Check sheet for the modelled part. Datum: model origin and axes. Units: mm. Coordinates: 2 decimals unless noted, no trailing zeros. Loops run counter-clockwise (first coordinate to the right, second up) from the corner with the lowest first, then second, coordinate; pieces in that order, holes last. Notation, with made-up numbers: M 21,56 L 80,56 A24 cw 80,72 Z; hole C -22,11 d9. An arc over 180 degrees is marked long. Return JSON: item names as keys, results as strings.
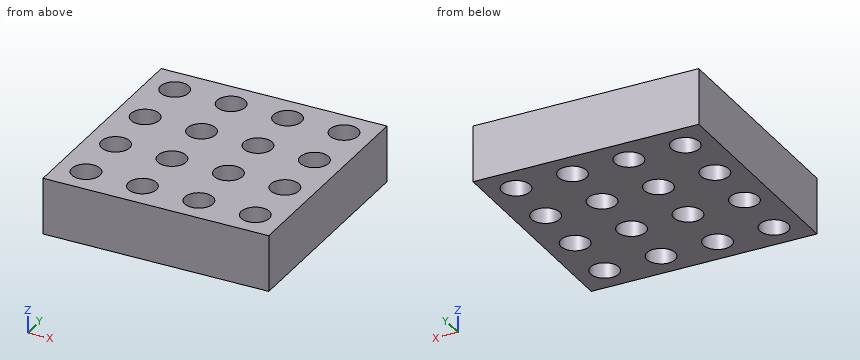
from build123d import *

# Parameters (mm, degrees)
SKETCH1_W            = 40
SKETCH1_H            = 40
BOSS_EXTRUDE1_DEPTH  = 10
SKETCH3_R            = 2.5
CUT_EXTRUDE1_DEPTH   = 11
LPATTERN1_COUNT      = 4
LPATTERN1_PITCH      = 10
LPATTERN1_COUNT_DIR2 = 4
LPATTERN1_PITCH_DIR2 = 10


with BuildPart() as part:
    # Sketch1 → Boss-Extrude1 (new body)
    with BuildSketch(Plane.XY):
        Rectangle(SKETCH1_W, SKETCH1_H)
    extrude(amount=BOSS_EXTRUDE1_DEPTH)

    # Sketch3 → Cut-Extrude1 (cut, through all)
    with BuildSketch(Plane.XY.offset(10)):
        with Locations((15, 15)):
            Circle(SKETCH3_R)
    cut_extrude1 = extrude(amount=-CUT_EXTRUDE1_DEPTH, mode=Mode.SUBTRACT)

    # LPattern1: Cut-Extrude1 4 × 4
    with Locations(*[(-i * LPATTERN1_PITCH, -j * LPATTERN1_PITCH_DIR2, 0) for i in range(LPATTERN1_COUNT) for j in range(LPATTERN1_COUNT_DIR2) if (i, j) != (0, 0)]):
        add(cut_extrude1, mode=Mode.SUBTRACT)


solid = part.part
1) Section check B-B on z = 3.25. Count the separate pieces of the cut face and the enclosed holes in it, then the cut area to 3 significant figures.
Answers:
{"separate pieces": "1", "enclosed holes": "16", "area": "1,290 mm²"}
2) Scan lines: line 1 along Y through (x, z) = (5, 6); line 2 along Y through (x, z) = (4, 2.5); line 3 along X through (y, z) = (-13, 4.5). Record each from-to range of solid material in increasing order. Write a range as [from, to].
Answers:
{"line 1": "[-20, -17.5], [-12.5, -7.5], [-2.5, 2.5], [7.5, 12.5], [17.5, 20]", "line 2": "[-20, -17.29], [-12.71, -7.29], [-2.71, 2.71], [7.29, 12.71], [17.29, 20]", "line 3": "[-20, -16.5], [-13.5, -6.5], [-3.5, 3.5], [6.5, 13.5], [16.5, 20]"}
3) Go/stop test with flat-tipped pins: pin 1 Ø6 at (x, y) = (15, -15) entering from +Z; pin 2 Ø4.5 at (x, y) = (-5, 15) entering from +Z. Record where each tip stops, or that it passes through.
Answers:
{"pin 1": "z = 10", "pin 2": "through"}
4) Section check A-A on x = 15. Record the cut outline in (y, z).
Answers:
{"outline": "M -20,0 L -17.5,0 L -17.5,10 L -20,10 Z; M -12.5,0 L -7.5,0 L -7.5,10 L -12.5,10 Z; M -2.5,0 L 2.5,0 L 2.5,10 L -2.5,10 Z; M 7.5,0 L 12.5,0 L 12.5,10 L 7.5,10 Z; M 17.5,0 L 20,0 L 20,10 L 17.5,10 Z"}
5) Section check C-C on y = 6.5. Record the cut outline in (x, z).
Answers:
{"outline": "M -20,0 L -17,0 L -17,10 L -20,10 Z; M -13,0 L -7,0 L -7,10 L -13,10 Z; M -3,0 L 3,0 L 3,10 L -3,10 Z; M 7,0 L 13,0 L 13,10 L 7,10 Z; M 17,0 L 20,0 L 20,10 L 17,10 Z"}
